```python
from build123d import *

# Parameters (mm, degrees)
EXTRUDE_1_DEPTH     = 12
SKETCH_2_R          = 1
CUT_EXTRUDE_1_DEPTH = 4
SKETCH_3_R          = 1
CUT_EXTRUDE_2_DEPTH = 10


with BuildPart() as part:
    # 草图1 → 凸台-拉伸1 (new body)
    with BuildSketch(Plane.XY):
        with BuildLine():
            Line((0, 8), (4.9, 8))
            Line((4.9, 8), (4.9, 25.5))
            Line((4.9, 25.5), (8.9, 25.5))
            Line((8.9, 25.5), (8.9, -48.754024521))
            Line((8.9, -48.754024521), (4.9, -48.754024521))
            Line((4.9, -48.754024521), (0, -48))
            ThreePointArc((0, -48), (-4.07207787, -46.886086103), (-7.010169708, -43.854545455))
            ThreePointArc((-7.010169708, -43.854545455), (-8.111954148, -42.717717711), (-9.638983349, -42.3))
            Line((-9.638983349, -42.3), (-12.681165581, -42.3))
            Line((-12.681165581, -42.3), (-12.681165581, -40.3))
            Line((-12.681165581, -40.3), (-4.990991885, -40.3))
            ThreePointArc((-4.990991885, -40.3), (5, -40), (-4.990991885, -39.7))
            Line((-4.990991885, -39.7), (-12.681165581, -39.7))
            Line((-12.681165581, -39.7), (-12.681165581, -37.7))
            Line((-12.681165581, -37.7), (-9.638983349, -37.7))
            ThreePointArc((-9.638983349, -37.7), (-8.111954148, -37.282282289), (-7.010169708, -36.145454545))
            ThreePointArc((-7.010169708, -36.145454545), (-4.07207787, -33.113913897), (0, -32))
            Line((0, -32), (4.9, -32))
            Line((4.9, -32), (4.9, -31))
            Line((4.9, -31), (4.9, -8.754024521))
            Line((4.9, -8.754024521), (0, -8))
            ThreePointArc((0, -8), (-4.07207787, -6.886086103), (-7.010169708, -3.854545455))
            ThreePointArc((-7.010169708, -3.854545455), (-8.111954148, -2.717717711), (-9.638983349, -2.3))
            Line((-9.638983349, -2.3), (-12.681165581, -2.3))
            Line((-12.681165581, -2.3), (-12.681165581, -0.3))
            Line((-12.681165581, -0.3), (-4.990991885, -0.3))
            ThreePointArc((-4.990991885, -0.3), (5, 0), (-4.990991885, 0.3))
            Line((-4.990991885, 0.3), (-12.681165581, 0.3))
            Line((-12.681165581, 0.3), (-12.681165581, 2.3))
            Line((-12.681165581, 2.3), (-9.638983349, 2.3))
            ThreePointArc((-9.638983349, 2.3), (-8.111954148, 2.717717711), (-7.010169708, 3.854545455))
            ThreePointArc((-7.010169708, 3.854545455), (-4.07207787, 6.886086103), (0, 8))
        make_face()
    extrude(amount=EXTRUDE_1_DEPTH)

    # 草图2 → 切除-拉伸1 (cut)
    with BuildSketch(Plane.ZY.offset(-4.9)):
        with Locations((6, 22.5)):
            Circle(SKETCH_2_R)
        with Locations((6, -23.78)):
            Circle(SKETCH_2_R)
    extrude(amount=-CUT_EXTRUDE_1_DEPTH, mode=Mode.SUBTRACT)

    # 草图3 → 切除-拉伸2 (cut)
    with BuildSketch(Plane(origin=(0, 2.3, 0), x_dir=(1, 0, 0), z_dir=(0, 1, 0))):
        with Locations((-11.081165581, -6)):
            Circle(SKETCH_3_R)
    extrude(amount=-CUT_EXTRUDE_2_DEPTH, mode=Mode.SUBTRACT)


solid = part.part
```
Model file for the job. Use its own axes, mm. A direction names the side the tool comes from. Coordinates: 2 decimals unless noted, no trailing zeros. Write each loop counter-clockwise with the first axis right and the second up, starting at its lowest first coordinate (ties: lowest second). Pieces come first, ordered by that corner, then holes. Notation, with made-up numbers: (2.5, 84.25) - (47.5, 84.25) arc R29 cw to (47.5, 119.25) - close; hole circle Ø1 at (72.5, 58.25). An arc over 180 degrees is marked (long way). Use a Markdown table: item, result. Add a question column.
Item 1: Band-saw the part on D-D, the plane y = 10. Write the cut outline in (x, z), and give its area (3 significant figures).
Item 2: Drop flat-ended pins along their axis: pin 1 (6 mm diameter, centred on x = -9.5, z = 3.5, fed in from -Y); pin 2 (3.5 mm diameter, centred on y = 14, z = 6.5, fed in from -X); pin 3 (3 mm diameter, centred on x = -11.08, z = 6, fed in from -Y). Give the stop position or say it passes through.
Item 3: Band-saw the part on A-A, the plane y = 22.5. Write the cut outline in (x, z), and give its area (3 significant figures).
Item 4: Band-saw the part on B-B, the plane x = -1.75. Write the cut outline in (y, z).
Item 5: Two-plate mould, pull along Z, no slides. Class faces 1 (the face through (5.5, -11.1, 12)), 2 (the face through (6.872, 21.524, 5.783)), 3 (the face through (-8.131, -37.294, 5.916)): pulls with the +Z half, pulls with the -Z half, needs draft (parallel to the pull), parting line crosses it, or undercut.
Item 6: Drill centre lines: line 1 along Y through (x, z) = (-9.5, 10.75); line 2 along Y through (x, z) = (8, 6); line 3 along Y through (x, z) = (-0.25, 1). Where is each one in solid material? Low to high.
Item 7: 3-axis set-ups, long thin cutter, end or side, ignore diameter. For faces 4 (the face through (-8.09, -2.73, 5.92)), 5 (the face through (-10.127, 1.314, 5.7)), 6 (the face through (4.9, 17, 6)), 7 (the face through (-11, -42.3, 6)): which of +Z, -Z, +X, -X, +Y, -Y reach the whole face in a straight line?
A:
| question | item | result |
|---|---|---|
| 1 | outline | (4.9, 0) - (8.9, 0) - (8.9, 12) - (4.9, 12) - close |
| 1 | area | 48.0 mm² |
| 2 | pin 1 | stops at y = -44.66 |
| 2 | pin 2 | stops at x = 4.9 |
| 2 | pin 3 | stops at y = -42.3 |
| 3 | outline | (4.9, 0) - (8.9, 0) - (8.9, 5) - (4.9, 5) - close; (4.9, 7) - (8.9, 7) - (8.9, 12) - (4.9, 12) - close |
| 3 | area | 40.0 mm² |
| 4 | outline | (-47.81, 0) - (-44.68, 0) - (-44.68, 12) - (-47.81, 12) - close; (-35.32, 0) - (-32.19, 0) - (-32.19, 12) - (-35.32, 12) - close; (-7.81, 0) - (-4.68, 0) - (-4.68, 12) - (-7.81, 12) - close; (4.68, 0) - (7.81, 0) - (7.81, 12) - (4.68, 12) - close |
| 5 | face 1 | pulls with the +Z half |
| 5 | face 2 | undercut |
| 5 | face 3 | needs draft |
| 6 | line 1 | y = -42.3 to -40.3, -39.7 to -37.7, -2.3 to -0.3, 0.3 to 2.3 |
| 6 | line 2 | y = -48.75 to -24.78, -22.78 to 21.5, 23.5 to 25.5 |
| 6 | line 3 | y = -48 to -44.99, -35.01 to -32, -8 to -4.99, 4.99 to 8 |
| 7 | face 4 | +Z, -Z, -X |
| 7 | face 5 | +Y |
| 7 | face 6 | +Z, -Z, -X, +Y |
| 7 | face 7 | +Z, -Z, -X, -Y |
